Autodesk Fusion 360 part; units mm, degrees
sketch "Sketch1" plane through (0, 0, 0) normal (0, 1, 0) x (1, 0, 0)
  line L0 (-38.1, 0) -> (0, 0)
  line L1 (0, 0) -> (0, -38.1)
  line L2 (-38.1, -1.5875) -> (-1.5875, -1.5875)
  line L3 (-1.5875, -1.5875) -> (-1.5875, -38.1)
  line L4 (-1.5875, -38.1) -> (0, -38.1)
  line L5 (-38.1, -1.5875) -> (-38.1, 0)
  dimension "d5" = 38.1
  dimension "d6" = 1.5875
extrude "Extrude1" add sketch "Sketch1" along normal blind 400
sketch "Sketch3" plane through (-1.5875, 0, 0) normal (-1, 0, 0) x (0, -1, 0)
  line L0 (0, 1.5875) -> (0, 38.1)
  line L1 (0, 38.1) -> (-400, 38.1)
  line L2 (-400, 38.1) -> (-400, 1.5875)
  line L3 (-400, 1.5875) -> (0, 1.5875)
  circle A0 centre (-392, 10) radius 4.9317
  circle A1 centre (-8, 20) radius 5
  line L4 (0, 0) -> (-400, 0)
  dimension "d15" = 10
  dimension "d16" = 8
  dimension "d17" = 8
  dimension "d18" = 20
hole "Hole2" at (-1.5875, 8, 20) at (-1.5875, 392, 10) direction (1, 0, 0) diameter 5.5 depth 7 tip angle 118
sketch "Sketch4" plane through (0, 0, 1.5875) normal (0, 0, 1) x (-1, 0, 0)
  line L0 (38.1, 0) -> (1.5875, 0)
  line L1 (1.5875, 0) -> (1.5875, -400)
  line L2 (1.5875, -400) -> (38.1, -400)
  line L3 (38.1, -400) -> (38.1, 0)
  circle A0 centre (19.8375, -34.285) radius 6.9462
  circle A1 centre (19.8375, -365.715) radius 6.9462
  dimension "d22" = 34.285
  dimension "d23" = 34.285
  dimension "d24" = 18.25
hole "Hole3" at (-19.8375, 34.285, 1.5875) at (-19.8375, 365.715, 1.5875) direction (0, 0, -1) diameter 5.5 depth 7 tip angle 118
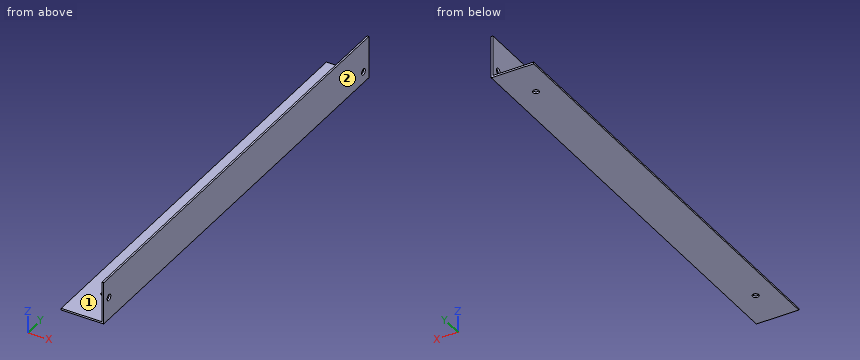
Geometry: final body of the model. Coordinates: model frame, mm. Face numbers are marked on the shaded views. A direction names the side the tool comes from. Round coordinates to 2 decimals unless told otherwise and drop trailing zeros. Loops run counter-clockwise (first coordinate to the right, second up) from the corner with the lowest first, then second, coordinate; pieces in that order, holes last. Notation, with made-up numbers: M 5,32 L 56,32 A29 cw 56,70 Z; hole C 70.5,35 d4. An arc over 180 degrees is marked long. Put each result on its own line as item: value. Start each with the question number.
(1) Set-up query: the marked faces 1 and 2. Return all of +Z, -Z, +X, -X, +Y, -Y with unobstructed straight access to the full face (end or side cutting, diameter ignored); none if empty.
(2) Section query C-C (x = -8.5). Return loops of the section in (y, z), then the cut area to 3 significant figures.
(3) Contact query for flat-ended pins moving along their axis: pin 1 Ø4 at (y, z) = (189, 23.5) entering from -X; pin 2 Ø3.5 at (y, z) = (392, 10) entering from -X. Output: stop coordinate, or through.
(4) Material intervals for line 1 along Y through (x, z) = (-0.45, 20); line 2 along Z through (x, y) = (-0.95, 8); line 3 along Z through (x, y) = (-0.7, 392), sorted ascending. Write a range as [from, to].
(5) Section query A-A (y = 195). Return loops of the section in (x, z), then the cut area to 3 significant figures.
(6) Section query B-B (z = 33.5). Return loops of the section in (x, y), then the cut area to 3 significant figures.
Findings below:
1. face 1: +Z, -X, +Y, -Y
1. face 2: +Z, -Z, +X, +Y, -Y
2. outline: M 0,0 L 400,0 L 400,1.59 L 0,1.59 Z
2. area: 635 mm2
3. pin 1: stops at x = -1.59
3. pin 2: passes through
4. line 1: y = [0, 5.25], [10.75, 400]
4. line 2: z = [0, 17.25], [22.75, 38.1]
4. line 3: z = [0, 7.25], [12.75, 38.1]
5. outline: M -38.1,0 L 0,0 L 0,38.1 L -1.59,38.1 L -1.59,1.59 L -38.1,1.59 Z
5. area: 118 mm2
6. outline: M -1.59,0 L 0,0 L 0,400 L -1.59,400 Z
6. area: 635 mm2
